Design review of the part built by this model. Coordinates are the model's own, in mm. A direction names the side the tool comes from. Coordinates: 2 decimals unless noted, no trailing zeros. Loops run counter-clockwise (first coordinate to the right, second up) from the corner with the lowest first, then second, coordinate; pieces in that order, holes last. Notation, with made-up numbers: (-4, -32) - (44, -32) arc R13 ccw to (44, -13) - close; hole circle Ø10 at (61, 28). An arc over 180 degrees is marked (long way). Answer in a Markdown table with one row per item. Add a question column.
(1) We need section B-B, the plane x = 6.5. Write out the cut boundary in (y, z).
(2) We need section C-C, the plane y = 0. Write out the cut boundary in (x, z).
(3) To check wall thickness, follow L1, parallel to Y at x = 0, z = -120; L2, parallel to Y at x = -0.5, z = -99; L3, parallel to Y at x = -15.5, z = -104. State the ranges of each line that lie inside material, in increasing order. Write a range as [from, to].
(4) The part is to be moulded in two halves that separate along Y. For faces 6 (the face through (0, -102, -122)), 7 (the face through (-23.648, -58.137, -122.362)), 8 (the face through (33.81, 11.02, -93.49)), say which applies: released by +Y, released by -Y, zero draft, split by the parting line, or undercut.
(5) We need section D-D, the plane y = -29. Write out the cut boundary in (x, z).
(6) For faces 1 (the face through (31.617, -8.307, -107.603)), 2 (the face through (23.648, -58.137, -122.362)), 3 (the face through (12.154, 33.392, -110.561)), 4 (the face through (-33.81, -11.02, -93.49)), 5 (the face through (38, 0, -115.292)), list the 3-axis set-ups (+Z, -Z, +X, -X, +Y, -Y) from which the entire face can be reached by the end or side of a thin tool; tool diameter is ignored.
(7) Clearance check with flat-ended pins moving along their axes: pin 1 (3 mm diameter, centred on x = -34, z = -114, fed in from +Y); pin 2 (1.7 mm diameter, centred on x = 37.5, z = -106.5, fed in from +Y); pin 3 (12 mm diameter, centred on x = -30, z = -112.5, fed in from +Y). State where each tip first meets the part, or that it passes through.
(8) We need section A-A, the plane z = -101.5. Write out the cut boundary in (x, y).
from build123d import *

# Parameters (mm, degrees)
SKETCH022_R        = 40
SKETCH022_R_2      = 31
PAD006_DEPTH       = 33
SKETCH023_W        = 90
SKETCH023_H        = 14
POCKET010_DEPTH    = 21
CHAMFER_SIZE       = 6
POCKET011_DEPTH    = 268.7042032027
POLARPATTERN_COUNT = 2
FILLET001_R        = 8
PAD008_DEPTH       = 5
SKETCH028_R        = 1.5
POCKET013_DEPTH    = 3.5
SKETCH029_R        = 2
PAD009_DEPTH       = 10


with BuildPart() as part:
    # Sketch022 (on DatumPlane) → Pad006 (new body)
    with BuildSketch(Plane.XY.offset(-127.29162)):
        Circle(SKETCH022_R)
        Circle(SKETCH022_R_2, mode=Mode.SUBTRACT)
    extrude(amount=PAD006_DEPTH)

    # Sketch023 (on Face4 of Pad006) → Pocket010 (cut)
    with BuildSketch(Plane.XY.offset(-94.29162)):
        Rectangle(SKETCH023_W, SKETCH023_H)
    extrude(amount=-POCKET010_DEPTH, mode=Mode.SUBTRACT)

    # Chamfer
    chamfer_edges = [part.edges().sort_by_distance(p)[0] for p in [
        (-31, 0, -115.29162),
        (30.799184, -3.522821, -115.29162),
    ]]
    chamfer(chamfer_edges, length=CHAMFER_SIZE)

    # Sketch024 (on Face8 of Chamfer) → Pocket011 (cut, through all)
    with BuildSketch(Plane.XY.offset(-94.29162)):
        with BuildLine():
            ThreePointArc((-32.9089653438, -19), (-24.4259291681, -29.1096888385), (-12.9967654464, -35.7083195899))
            Line((-12.9967654464, -35.7083195899), (-11.2866647297, -31.0098564859))
            ThreePointArc((-28.5788383249, -16.5), (-21.2119911197, -25.2794666229), (-11.2866647297, -31.0098564859))
            Line((-32.9089653438, -19), (-28.5788383249, -16.5))
        make_face()
    pocket011 = extrude(amount=-POCKET011_DEPTH, mode=Mode.SUBTRACT)

    # PolarPattern: Pocket011 ×2 about axis
    polarpattern_axis = Axis((0, 0, -94.29162), (0, 0, 1))
    for i in range(1, POLARPATTERN_COUNT):
        add(pocket011.rotate(polarpattern_axis, i * 360 / POLARPATTERN_COUNT), mode=Mode.SUBTRACT)

    # Fillet001
    fillet001_edges = [part.edges().sort_by_distance(p)[0] for p in [
        (-30.199338, 7, -104.79162),
        (30.199338, -7, -104.79162),
    ]]
    fillet(fillet001_edges, radius=FILLET001_R)

    # Sketch027 (on Face7 of Fillet001) → Pad008 (join)
    with BuildSketch(Plane.XY.offset(-94.29162)):
        with BuildLine():
            ThreePointArc((-30.1993377411, -7), (-29.8652589516, -8.3106141622), (-29.4743299443, -9.6054085979))
            Line((-38.0313934765, -12.3940756103), (-29.4743299443, -9.605408598))
            ThreePointArc((-38.9668874079, -9.0322580645), (-38.5358180021, -10.7233731125), (-38.0313934765, -12.3940756103))
            Line((-38.9668874078, -9.0322580645), (-30.1993377411, -7))
        make_face()
        with BuildLine():
            Line((30.1993377411, 7), (38.9668874078, 9.0322580645))
            ThreePointArc((38.9668874078, 9.0322580645), (38.5358180021, 10.7233731125), (38.0313934765, 12.3940756102))
            Line((38.0313934765, 12.3940756103), (29.4743299443, 9.605408598))
            ThreePointArc((30.1993377411, 7), (29.8652589516, 8.3106141622), (29.4743299443, 9.6054085979))
        make_face()
    extrude(amount=PAD008_DEPTH)

    # Sketch028 (on Face20 of Pad008) → Pocket013 (cut, symmetric)
    with BuildSketch(Plane(origin=(0, 0, -127.29162), x_dir=(0.9507848369, 0.3098518903, 0), z_dir=(0.3098518903, -0.9507848369, 0))):
        with Locations((-35.5, 35.5)):
            Circle(SKETCH028_R)
        with Locations((35.5, 35.5)):
            Circle(SKETCH028_R)
    extrude(amount=POCKET013_DEPTH, both=True, mode=Mode.SUBTRACT)

    # Sketch029 (on Face19 of Pocket013) → Pad009 (join)
    with BuildSketch(Plane(origin=(0, 0, -127.29162), x_dir=(1, 0, 0), z_dir=(0, 0, -1))):
        with BuildLine():
            ThreePointArc((9.5394034408, 102.9999636655), (3e-10, 110), (-9.5394034406, 102.9999636661))
            Line((-9.5394034406, 102.9999636661), (-38.1575696347, 11.9999949821))
            ThreePointArc((38.1575696236, 11.9999950176), (-1.86e-08, 40), (-38.1575696347, 11.9999949821))
            Line((9.5394034408, 102.9999636656), (38.1575696236, 11.9999950176))
        make_face()
        with Locations((0, 100)):
            Circle(SKETCH029_R, mode=Mode.SUBTRACT)
    extrude(amount=-PAD009_DEPTH)


solid = part.part
Responses:
| question | item | result |
|---|---|---|
| 1 | outline | (-107.6, -127.29) - (-30.31, -127.29) - (-30.31, -94.29) - (-39.47, -94.29) - (-39.47, -117.29) - (-107.6, -117.29) - close; (30.31, -127.29) - (39.47, -127.29) - (39.47, -94.29) - (30.31, -94.29) - close |
| 2 | outline | (-40, -127.29) - (-31, -127.29) - (-31, -121.29) - (-37, -115.29) - (-40, -115.29) - close; (31, -127.29) - (40, -127.29) - (40, -115.29) - (37, -115.29) - (31, -121.29) - close |
| 3 | L1 | y = [-110, -102], [-98, -31], [31, 40] |
| 3 | L2 | y = [-40, -31], [31, 40] |
| 3 | L3 | y = [-36.87, -34.7], [-29.13, -26.85], [26.85, 36.87] |
| 4 | face 6 | undercut |
| 4 | face 7 | released by -Y |
| 4 | face 8 | released by +Y |
| 5 | outline | (-32.81, -127.29) - (-24.56, -127.29) - (-24.56, -94.29) - (-27.55, -94.29) - (-27.55, -117.29) - (-32.81, -117.29) - close; (-15.75, -127.29) - (-10.95, -127.29) - (-10.95, -94.29) - (-15.75, -94.29) - close; (10.95, -127.29) - (32.81, -127.29) - (32.81, -117.29) - (27.55, -117.29) - (27.55, -94.29) - (10.95, -94.29) - close |
| 6 | face 1 | +Z |
| 6 | face 2 | +Z, -Z, +X, -Y |
| 6 | face 3 | +Z, -Z |
| 6 | face 4 | +Z, +X, -Y |
| 6 | face 5 | +Z, +X, -X |
| 7 | pin 1 | stops at y = 23.32 |
| 7 | pin 2 | stops at y = 16.02 |
| 7 | pin 3 | stops at y = 32 |
| 8 | outline | (-39.38, -7) arc R40 ccw to (39.38, -7) - (36, -7) arc R8 ccw to (28.62, -11.92) arc R31 cw to (-30.2, -7) - close; (-39.38, 7) - (-36, 7) arc R8 ccw to (-28.62, 11.92) arc R31 cw to (30.2, 7) - (39.38, 7) arc R40 ccw to start; hole (-32.91, -19) arc R38 ccw to (-13, -35.71) - (-11.29, -31.01) arc R33 cw to (-28.58, -16.5) - close; hole (11.29, 31.01) arc R33 cw to (28.58, 16.5) - (32.91, 19) arc R38 ccw to (13, 35.71) - close |
